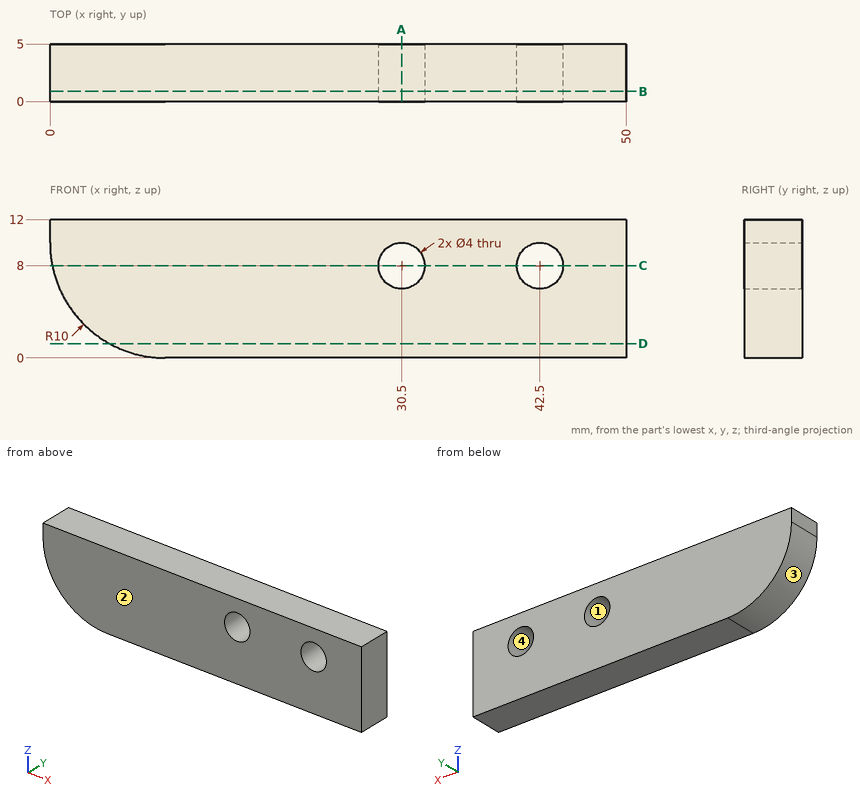
Could you check a few things on this drawing? It's one solid part, dimensions in mm from its lowest x, y, z. Coordinates: 2 decimals unless noted, no trailing zeros. Order: outer loops, then holes, each group sorted by start corner. A loop starts at its lowest first (then second) coordinate and runs counter-clockwise, first axis right, second up. Notation, with made-up numbers: (-29, 89.5) - (23, 89.5) arc R23 cw to (23, 124.5) - close; hole circle Ø4 at (-26.75, -25.75). An arc over 180 degrees is marked (long way). Answer as a JSON object with one key per item and string values. Group by question number.
Q1. I need wall thicknesses on line 1 (Z direction, x = 42.5, y = 2.5); line 2 (X direction, y = 2.7, z = 7.5); line 3 (X direction, y = 3.25, z = 8). Which ranges of each line are inside material? Lowest first, please. Write a range as from..to.
Q2. We'd pull the mould along X, two halves only. Please class the marked faces 1, 2, 3 and 4: +X half, -X half, draft (parallel to the pull), parting line (faces both ways), or undercut.
Q3. Will these pins go through, and if not, where does the flat tip stop? P1, Ø3, axis at x = 30.5, z = 8, coming from the -Y side; P2, Ø3, axis at y = 1.5, z = 4.5, coming from the -X side.
Q4. Imagine slicing it at B-B (y = 0.9). Please give me the cut outline in (x, z), and give its area (3 significant figures).
Q5. Imagine slicing it at C-C (z = 8). Please give me the cut outline in (x, y).
Q6. Imagine slicing it at A-A (x = 30.5). Please give me the cut outline in (y, z).
Q7. Imagine slicing it at D-D (z = 1.25). Please give me the cut outline in (x, y).
Determined:
{
 "1": {"line 1": "z = 0..6, 10..12", "line 2": "x = 0.32..28.56, 32.44..40.56, 44.44..50", "line 3": "x = 0.2..28.5, 32.5..40.5, 44.5..50"},
 "2": {"face 1": "undercut", "face 2": "draft", "face 3": "-X half", "face 4": "undercut"},
 "3": {"P1": "passes through", "P2": "stops at x = 0.83"},
 "4": {"outline": "(0, 10) arc R10 ccw to (10, 0) - (50, 0) - (50, 12) - (0, 12) - close; hole circle Ø4 at (30.5, 8); hole circle Ø4 at (42.5, 8)", "area": "553 mm2"},
 "5": {"outline": "(0.2, 0) - (28.5, 0) - (28.5, 5) - (0.2, 5) - close; (32.5, 0) - (40.5, 0) - (40.5, 5) - (32.5, 5) - close; (44.5, 0) - (50, 0) - (50, 5) - (44.5, 5) - close"},
 "6": {"outline": "(0, 0) - (5, 0) - (5, 6) - (0, 6) - close; (0, 10) - (5, 10) - (5, 12) - (0, 12) - close"},
 "7": {"outline": "(5.16, 0) - (50, 0) - (50, 5) - (5.16, 5) - close"}
}
